Verification items for the finished model (mm, model axes). A direction names the side the tool comes from. Round coordinates to 2 decimals unless told otherwise and drop trailing zeros. Order: outer loops, then holes, each group sorted by start corner. A loop starts at its lowest first (then second) coordinate and runs counter-clockwise, first axis right, second up. Notation, with made-up numbers: (4.25, 59) -> (51.25, 59) arc R28 cw to (51.25, 86) -> close; hole circle Ø2 at (-5, -27). An arc over 180 degrees is marked (long way). Put each result on its own line as item: value.
Autodesk Inventor part; units mm, degrees
ref_plane "YZ Plane" through (0, 0, 0) normal (1, 0, 0) x (0, 1, 0)
ref_plane "XZ Plane" through (0, 0, 0) normal (0, 1, 0) x (-1, 0, 0)
ref_plane "XY Plane" through (0, 0, 0) normal (0, 0, 1) x (1, 0, 0)
sketch "Sketch1" plane through (0, 0, 0) normal (0, 0, 1) x (1, 0, 0)
  circle A0 centre (0, 0) radius 4
  dimension "d0" = 8
extrude "Extrusion1" add sketch "Sketch1" along normal blind 6
sketch "Sketch2" plane through (0, 0, 6) normal (0, 0, 1) x (1, 0, 0)
  line L0 (2.1, 1.125) -> (2.5, 1.125)
  line L1 (2.5, 1.125) -> (2.5, -1.125)
  line L2 (2.5, -1.125) -> (2.1, -1.125)
  line L3 (2.1, -1.125) -> (2.1, 1.125)
  line L4 (-2.5, 1.125) -> (-2.1, 1.125)
  line L5 (-2.1, 1.125) -> (-2.1, -1.125)
  line L6 (-2.1, -1.125) -> (-2.5, -1.125)
  line L7 (-2.5, -1.125) -> (-2.5, 1.125)
  point P0 (0, 0)
  point P1 (2.1, 0)
  point P2 (-2.5, 0)
  dimension "d3" = 2.25
  dimension "d6" = 2.25
  dimension "d9" = 0.4
  dimension "d10" = 0.4
  dimension "d11" = 2.5
  dimension "d12" = 2.5
extrude "Extrusion2" add sketch "Sketch2" along normal blind 5.5
sketch "Sketch3" plane through (2.5, -1.125, 6) normal (1, 0, 0) x (0, 0, -1)
  line L0 (0, 2.25) -> (-5.5, 2.25)
  line L1 (0, 2.25) -> (-2.5, 2.25)
  arc A0 (-4.5, 2.25) -> (-2.5, 2.25) centre (-3.5, 3.549) ccw
  line L2 (-5.5, 0) -> (-5.5, 2.25)
  line L3 (-5.5, 1.125) -> (-5.2177, 1.125)
  arc A1 (-5.1597, 2.25) -> (-5.5, 1.9097) centre (-5.1597, 1.9097) ccw
  line L4 (-5.5, 1.9097) -> (-5.1597, 2.25) construction
  line L5 (-5.5, 1.9097) -> (-5.0187, 1.9097) construction
  line L6 (-5.5, 1.125) -> (-5.5, 1.9097)
  line L7 (-5.1597, 2.25) -> (-4.5, 2.25)
  arc A2 (-2.5, 0) -> (-4.5, 0) centre (-3.5, -1.299) ccw
  arc A3 (-5.5, 0.3403) -> (-5.1597, 0) centre (-5.1597, 0.3403) ccw
  line L8 (0, 0) -> (-5.5, 0)
  line L9 (-5.5, 0.3403) -> (-5.5, 0)
  line L10 (-5.5, 0) -> (-5.1597, 0)
  line L11 (-4.5, 0) -> (-2.5, 0)
  point P0 (6, 1.125)
  dimension "d15" = 2.5
  dimension "d16" = 2
  dimension "d17" = 45
extrude "Extrusion3" cut sketch "Sketch3" against normal up to surface (5 mm away)
sketch "Sketch4" plane through (0, 0, 0) normal (0, 1, 0) x (-1, 0, 0)
  line L0 (0, 0) -> (0, -3.2)
  line L1 (0, -3.2) -> (5, -3.2)
  line L2 (5, -3.2) -> (5, -1.4)
  line L3 (-4, 0) -> (4, 0)
  arc A0 (5, -1.4404) -> (4, 0) centre (3.4626, -1.4404) ccw
  line L4 (4, 0) -> (0, 0)
  dimension "d20" = 3.2
  dimension "d21" = 5
  dimension "d22" = 1.8
revolve "Revolution1" add sketch "Sketch4" angle 360 about axis through (0, 0, 0) along (0, 0, -1)
sketch "Sketch5" plane through (0, 0, -3.2) normal (0, 0, -1) x (-1, 0, 0)
  circle A0 centre (0, 0) radius 3.5
  dimension "d24" = 7
extrude "Extrusion4" add sketch "Sketch5" along normal blind 1.5
sketch "Sketch7" plane through (0, 0, -4.7) normal (0, 0, -1) x (-1, 0, 0)
  circle A0 centre (0, 0) radius 3.525
  dimension "d29" = 7.05
extrude "Extrusion6" add sketch "Sketch7" along normal blind 5
thread "Thread1"
sketch "Sketch8" plane through (0, 0, -9.7) normal (0, 0, -1) x (-1, 0, 0)
  circle A0 centre (0, 0) radius 2
  dimension "d34" = 4
extrude "Extrusion7" add sketch "Sketch8" along normal blind 3
sketch "Sketch9" plane through (0, 0, -12.7) normal (0, 0, -1) x (-1, 0, 0)
  circle A0 centre (0, 0) radius 3
  dimension "d37" = 6
extrude "Extrusion8" add sketch "Sketch9" along normal blind 3
fillet "Fillet1" radius 0.5 2 edges at (3, 0, -12.7) (3, 0, -15.7)
fillet "Fillet2" radius 0.2 1 edges at (-4, 0, 6)
equation "\"d9\" = d10"
properties part number "Push Button"
Item 1: Material ranges on line 1 along Z through (x, y) = (-1.5, -2.5); line 2 along Z through (x, y) = (-2, 2); line 3 along Z through (x, y) = (-3.75, 0), recorded low to high.
Geometry check:
line 1: -15.48 to -12.92, -9.7 to 6
line 2: -15.58 to -12.82, -9.7 to 6
line 3: -3.2 to 6
Item 2: Depth check by flat-ended pin: pin 1 Ø2 at (x, y) = (0.5, -0.5) entering from +Z; pin 2 Ø1.5 at (x, z) = (-3.5, 1) entering from +Y; pin 3 Ø1 at (x, z) = (1.5, 4) entering from +Y. Enter the tip coordinate at first touch or a pass-through.
Geometry check:
pin 1: z = 6
pin 2: y = 2.9
pin 3: y = 3.87
Item 3: Tool access check on faces 4 (the face through (-2.1, 0, 9)), 5 (the face through (3, 0, -14)), 6 (the face through (2.5, 0, 9)), 7 (the face through (1, 2, -12.7)), 8 (the face through (-2.5, 0, 9)). Record the directions out of +Z, -Z, +X, -X, +Y, -Y that give a thin tool (end or side, any length) a straight path to the whole face; none if there is none.
Geometry check:
face 4: +Z, +Y, -Y
face 5: -Z
face 6: +Z, +X, +Y, -Y
face 7: none
face 8: +Z, -X, +Y, -Y
Item 4: Sectioned sample at B-B, the plane z = -7.25. Record the boundary of the cut face in (x, y) (3 decimals).
Geometry check:
outline: circle Ø7.05 at (0, 0)
Item 5: Release check for a two-part mould opening along Z. For faces 1 (the face through (0, 2, -11)), 2 (the face through (-0.867, 3.905, 2.859)), 3 (the face through (0, 0, 6)) record: pulls with the +Z half, pulls with the -Z half, needs draft (parallel to the pull), parting line crosses it, or undercut.
Geometry check:
face 1: undercut
face 2: needs draft
face 3: pulls with the +Z half
Item 6: Sectioned sample at C-C, the plane z = 1. Record the boundary of the cut face in (x, y).
Geometry check:
outline: circle Ø8 at (0, 0)
